Could you check a few things on this model? Use its own coordinates, in mm. Give positions to 0.01 mm unless a question says otherwise; leave off trailing zeros. Loops run counter-clockwise (first coordinate to the right, second up) from the corner with the lowest first, then second, coordinate; pieces in that order, holes last. Notation, with made-up numbers: M 23.25,-3 L 58.25,-3 A16 ccw 58.25,1 Z; hole C 7.25,81 d11. An arc over 180 degrees is marked long. Use CSV: the item, a comma, the result in double quotes.
```python
from build123d import *

# Parameters (mm, degrees)
EXTRUDE_1_DEPTH      = 3
SKETCH_4_R           = 1.5
CUT_EXTRUDE_2_DEPTH  = 10
SKETCH_5_R           = 1.5
CUT_EXTRUDE_3_DEPTH  = 10
FILLET_1_R           = 5
SKETCH_6_W           = 116.747996977
SKETCH_6_H           = 25
SKETCH_6_W_2         = 124.073590325
SKETCH_6_W_3         = 98.220869454
SKETCH_6_W_4         = 117.634329044
CUT_EXTRUDE_4_DEPTH  = 10
SKETCH_7_W           = 65
SKETCH_7_H           = 110
CUT_EXTRUDE_5_DEPTH  = 10
FILLET_2_R           = 5
FILLET_3_R           = 5
SKETCH_9_R           = 6.308122895
CUT_EXTRUDE_7_DEPTH  = 10
SKETCH_10_R          = 1.5
CUT_EXTRUDE_8_DEPTH  = 10
SKETCH_11_R          = 1.5
CUT_EXTRUDE_9_DEPTH  = 10
SKETCH_12_W          = 120.586074841
SKETCH_12_H          = 63.347236109
SKETCH_12_W_2        = 131.774283424
SKETCH_12_H_2        = 66.604431946
CUT_EXTRUDE_10_DEPTH = 10
FILLET_4_R           = 10


with BuildPart() as part:
    # 草图2 → 凸台-拉伸1 (new body)
    with BuildSketch(Plane.XY):
        with BuildLine():
            Line((-16.583123952, 25), (0, 25))
            Line((0, 25), (0, 55))
            Line((0, 55), (91.6, 55))
            Line((91.6, 55), (91.6, 25))
            Line((91.6, 25), (108.183123952, 25))
            Line((108.183123952, 25), (188.183123952, 25))
            Line((188.183123952, 25), (188.183123952, 0))
            Line((188.183123952, 0), (91.6, 0))
            ThreePointArc((91.6, 0), (128.211652352, -88.388347648), (216.6, -125))
            Line((216.6, -125), (246.6, -125))
            Line((246.6, -125), (246.6, -215))
            Line((246.6, -215), (216.6, -215))
            ThreePointArc((216.6, -215), (128.211652352, -251.611652352), (91.6, -340))
            Line((91.6, -340), (188.183123952, -340))
            Line((188.183123952, -340), (188.183123952, -365))
            Line((188.183123952, -365), (108.183123952, -365))
            Line((108.183123952, -365), (91.6, -365))
            Line((91.6, -365), (91.6, -395))
            Line((91.6, -395), (0, -395))
            Line((0, -395), (0, -365))
            Line((0, -365), (-16.583123952, -365))
            Line((-16.583123952, -365), (-96.583123952, -365))
            Line((-96.583123952, -365), (-96.583123952, -340))
            Line((-96.583123952, -340), (0, -340))
            ThreePointArc((0, -340), (-36.611652352, -251.611652352), (-125, -215))
            Line((-125, -215), (-155, -215))
            Line((-155, -215), (-155, -125))
            Line((-155, -125), (-125, -125))
            ThreePointArc((-125, -125), (-36.611652352, -88.388347648), (0, 0))
            Line((0, 0), (-96.583123952, 0))
            Line((-96.583123952, 0), (-96.583123952, 25))
            Line((-96.583123952, 25), (-16.583123952, 25))
        make_face()
    extrude(amount=EXTRUDE_1_DEPTH)

    # 草图4 → 切除-拉伸2 (cut)
    with BuildSketch(Plane.XY.offset(3)):
        with Locations((-90.583123952, 20)):
            Circle(SKETCH_4_R)
        with Locations(Location((-90.583123952, 5, 0), (0, 0, 180))):
            Circle(SKETCH_4_R)
        with Locations((-90.583123952, -345)):
            Circle(SKETCH_4_R)
        with Locations(Location((-90.583123952, -360, 0), (0, 0, 180))):
            Circle(SKETCH_4_R)
        with Locations((182.183123952, -360)):
            Circle(SKETCH_4_R)
        with Locations(Location((182.183123952, -345, 0), (0, 0, 180))):
            Circle(SKETCH_4_R)
        with Locations((182.183123952, 5)):
            Circle(SKETCH_4_R)
        with Locations(Location((182.183123952, 20, 0), (0, 0, 180))):
            Circle(SKETCH_4_R)
    extrude(amount=-CUT_EXTRUDE_2_DEPTH, mode=Mode.SUBTRACT)

    # 草图5 → 切除-拉伸3 (cut)
    with BuildSketch(Plane.XY.offset(3)):
        with Locations((8, -10)):
            Circle(SKETCH_5_R)
        with Locations(Location((83.6, -10, 0), (0, 0, 180))):
            Circle(SKETCH_5_R)
        with Locations((83.6, -330)):
            Circle(SKETCH_5_R)
        with Locations(Location((8, -330, 0), (0, 0, 180))):
            Circle(SKETCH_5_R)
        with Locations((196.6, -135)):
            Circle(SKETCH_5_R)
        with Locations(Location((196.6, -205, 0), (0, 0, 180))):
            Circle(SKETCH_5_R)
        with Locations((-105, -205)):
            Circle(SKETCH_5_R)
        with Locations(Location((-105, -135, 0), (0, 0, 180))):
            Circle(SKETCH_5_R)
    extrude(amount=-CUT_EXTRUDE_3_DEPTH, mode=Mode.SUBTRACT)

    # 圆角1
    fillet_1_edges = [part.edges().sort_by_distance(p)[0] for p in [
        (-96.583123952, 0, 1.5),
        (-96.583123952, 25, 1.5),
        (0, 55, 1.5),
        (91.6, 55, 1.5),
        (188.183123952, 25, 1.5),
        (188.183123952, 0, 1.5),
        (246.6, -125, 1.5),
        (246.6, -215, 1.5),
        (188.183123952, -340, 1.5),
        (188.183123952, -365, 1.5),
        (91.6, -395, 1.5),
        (0, -395, 1.5),
        (-96.583123952, -365, 1.5),
        (-96.583123952, -340, 1.5),
        (-155, -215, 1.5),
        (-155, -125, 1.5),
    ]]
    fillet(fillet_1_edges, radius=FILLET_1_R)

    # 草图6 → 切除-拉伸4 (cut)
    with BuildSketch(Plane.XY.offset(3)):
        with Locations((-58.373998489, 12.5)):
            Rectangle(SKETCH_6_W, SKETCH_6_H)
        with Locations((153.636795163, 12.5)):
            Rectangle(SKETCH_6_W_2, SKETCH_6_H)
        with Locations((-49.110434727, -352.5)):
            Rectangle(SKETCH_6_W_3, SKETCH_6_H)
        with Locations((150.417164522, -352.5)):
            Rectangle(SKETCH_6_W_4, SKETCH_6_H)
    extrude(amount=-CUT_EXTRUDE_4_DEPTH, mode=Mode.SUBTRACT)

    # 草图7 → 切除-拉伸5 (cut)
    with BuildSketch(Plane.XY.offset(3)):
        with Locations((45.8, 55)):
            Rectangle(SKETCH_7_W, SKETCH_7_H)
        with Locations((45.8, -395)):
            Rectangle(SKETCH_7_W, SKETCH_7_H)
    extrude(amount=-CUT_EXTRUDE_5_DEPTH, mode=Mode.SUBTRACT)

    # 圆角2
    fillet_2_edges = [part.edges().sort_by_distance(p)[0] for p in [
        (13.3, 55, 1.5),
        (78.3, 55, 1.5),
        (78.3, -395, 1.5),
        (13.3, -395, 1.5),
    ]]
    fillet(fillet_2_edges, radius=FILLET_2_R)

    # 圆角3
    fillet_3_edges = [part.edges().sort_by_distance(p)[0] for p in [
        (13.3, 0, 1.5),
        (78.3, 0, 1.5),
        (78.3, -340, 1.5),
        (13.3, -340, 1.5),
    ]]
    fillet(fillet_3_edges, radius=FILLET_3_R)

    # 草图9 → 切除-拉伸7 (cut)
    with BuildSketch(Plane.XY.offset(3)):
        with Locations((228.308745857, -170)):
            Circle(SKETCH_9_R)
    extrude(amount=-CUT_EXTRUDE_7_DEPTH, mode=Mode.SUBTRACT)

    # 草图10 → 切除-拉伸8 (cut)
    with BuildSketch(Plane.XY.offset(3)):
        with Locations((-149, -149.5)):
            Circle(SKETCH_10_R)
        with Locations((-129, -149.5)):
            Circle(SKETCH_10_R)
        with Locations((-149, -190.5)):
            Circle(SKETCH_10_R)
        with Locations((-129, -190.5)):
            Circle(SKETCH_10_R)
    extrude(amount=-CUT_EXTRUDE_8_DEPTH, mode=Mode.SUBTRACT)

    # 草图11 → 切除-拉伸9 (cut)
    with BuildSketch(Plane.XY.offset(3)):
        with Locations((7.8, -114)):
            Circle(SKETCH_11_R)
        with Locations((83.8, -114)):
            Circle(SKETCH_11_R)
        with Locations((83.8, -226)):
            Circle(SKETCH_11_R)
        with Locations((7.8, -226)):
            Circle(SKETCH_11_R)
    extrude(amount=-CUT_EXTRUDE_9_DEPTH, mode=Mode.SUBTRACT)

    # 草图12 → 切除-拉伸10 (cut)
    with BuildSketch(Plane.XY.offset(3)):
        with Locations((60.293037421, 31.673618055)):
            Rectangle(SKETCH_12_W, SKETCH_12_H)
        with Locations((65.887141712, -373.302215973)):
            Rectangle(SKETCH_12_W_2, SKETCH_12_H_2)
    extrude(amount=-CUT_EXTRUDE_10_DEPTH, mode=Mode.SUBTRACT)

    # 圆角4
    fillet_4_edges = [part.edges().sort_by_distance(p)[0] for p in [
        (0, 0, 1.5),
        (91.6, 0, 1.5),
        (91.6, -340, 1.5),
        (0, -340, 1.5),
    ]]
    fillet(fillet_4_edges, radius=FILLET_4_R)


solid = part.part
```
1. I want a section at C-C, the plane x = -90. List the corners of the cut face in (y, z) for me.
Outcome:
outline,"M -220,0 L -120,0 L -120,3 L -220,3 Z"
2. I want a section at D-D, the plane y = -100. List the corners of the cut face in (x, z) for me, then the cut area to 3 significant figures.
Outcome:
outline,"M -50,0 L 141.6,0 L 141.6,3 L -50,3 Z"
area,"575 mm2"
3. I'm going to push flat-ended pins straight in: pin 1 Ø16.5 at (x, y) = (228.31, -170) entering from +Z; pin 2 Ø2.5 at (x, y) = (-149, -149.5) entering from -Z. Where does each tip first touch, or does it pass through?
Outcome:
pin 1,"z = 3"
pin 2,"through"
4. Please list where these lines run through material, in increasing order: line 1 (Y direction, x = -149, z = 1); line 2 (X direction, y = -330, z = 1.5); line 3 (Y direction, x = 8, z = 2.45).
Outcome:
line 1,"-215 to -192, -189 to -151, -148 to -125"
line 2,"-0.4 to 6.5, 9.5 to 82.1, 85.1 to 92"
line 3,"-339.87 to -331.5, -328.5 to -227.49, -224.51 to -115.49, -112.51 to -11.5, -8.5 to -0.13"
5. I want a section at B-B, the plane z = 1. Give the number of separate pieces and of enclosed holes in the cut face, then the cut area to 3 significant figures.
Outcome:
separate pieces,"1"
enclosed holes,"17"
area,"72,100 mm2"
6. I want a section at A-A, the plane y = -170. List the corners of the cut face in (x, z) for me, then the cut area to 3 significant figures.
Outcome:
outline,"M -155,0 L 222,0 L 222,3 L -155,3 Z; M 234.62,0 L 246.6,0 L 246.6,3 L 234.62,3 Z"
area,"1,170 mm2"
7. If we mould it in two halves opening along Y, with no side actions, what happens to faces 1 (the face through (132.513, -247.51, 1.479)), 2 (the face through (223.659, -165.737, 1.521)), 3 (the face through (49, -168, 3)), 4 (the face through (88.85, -2.74, 1.52))? For each: +Y half, -Y half, draft (parallel to the pull), parting line (faces both ways), or undercut.
Outcome:
face 1,"-Y half"
face 2,"undercut"
face 3,"draft"
face 4,"+Y half"
